Can you work these out from the model? Positions are in its coordinate system, mm. A direction names the side the tool comes from. Round coordinates to 2 decimals unless told otherwise and drop trailing zeros. Loops run counter-clockwise (first coordinate to the right, second up) from the corner with the lowest first, then second, coordinate; pieces in that order, holes last.
(1) I want a section at C-C on y = -7.5. Write out the boundary of the cut face in (x, z), plus the area to 3 significant figures.
(2) Which directions (+Z, -Z, +X, -X, +Y, -Y) give clear straight access to the entire face, cutting with the end or side of a thin tool? Please do faces 1 (the face through (0, 9, 6)), 2 (the face through (0, -9, -6)), 3 (the face through (4.93, -2.17, -9.76)), 4 (the face through (0, 0, 8)), 5 (the face through (0, 0, -8)).
(3) Will these pins go through, and if not, where does the flat tip stop? pin 1 Ø5 at (x, y) = (-61, -9) entering from -Z; pin 2 Ø6 at (y, z) = (-19, 7.5) entering from -X; pin 3 Ø4 at (y, z) = (17.5, 4.5) entering from -X.
(4) If I drill on line 1 along Z through (x, y) = (-55.5, 2); line 2 along X through (y, z) = (9.5, -3.25); line 3 along X through (y, z) = (-21.5, -5), over which ranges is the centre line in solid material (lowest first)?
(5) I want a section at D-D on x = -29. Write out the boundary of the cut face in (y, z).
(6) I want a section at B-B on z = 1.25. Write out the boundary of the cut face in (x, y), plus the area to 3 significant figures.
(7) I want a section at A-A on y = 0. Write out the boundary of the cut face in (x, z), plus the area to 3 significant figures.
from build123d import *

# Parameters (mm, degrees)
F0_R     = 10
F1_DEPTH = 10
F3_DEPTH = 7.5


with BuildPart() as f1:
    # F0 (on Right) → F1 (new body)
    with BuildSketch(Plane.YZ):
        Circle(F0_R)
    extrude(amount=F1_DEPTH)

    # F2 (on Top) → F3 (join, symmetric)
    with BuildSketch(Plane.XY):
        Polygon((-5, 25), (-65, 25), (-70, 10), (-70, -10), (-65, -25), (-5, -25), (0, -10), (0, 10), align=None)
    extrude(amount=F3_DEPTH, both=True)


solid = f1.part
Filled sheet:
1. outline: (-70, -7.5) - (0, -7.5) - (0, -6.61) - (10, -6.61) - (10, 6.61) - (0, 6.61) - (0, 7.5) - (-70, 7.5) - close
1. area: 1,180 mm2
2. face 1: +Z, +X, +Y
2. face 2: -Z, +X, -Y
2. face 3: +X
2. face 4: +Z, -X, +Y, -Y
2. face 5: -Z, -X, +Y, -Y
3. pin 1: stops at z = -7.5
3. pin 2: stops at x = -68
3. pin 3: stops at x = -68.17
4. line 1: z = -7.5 to 7.5
4. line 2: x = -70 to 0
4. line 3: x = -66.17 to -3.83
5. outline: (-25, -7.5) - (25, -7.5) - (25, 7.5) - (-25, 7.5) - close
6. outline: (-70, -10) - (-65, -25) - (-5, -25) - (0, -10) - (0, -9.92) - (10, -9.92) - (10, 9.92) - (0, 9.92) - (0, 10) - (-5, 25) - (-65, 25) - (-70, 10) - close
6. area: 3,550 mm2
7. outline: (-70, -7.5) - (0, -7.5) - (0, -10) - (10, -10) - (10, 10) - (0, 10) - (0, 7.5) - (-70, 7.5) - close
7. area: 1,250 mm2
